from build123d import *

# Parameters (mm, degrees)
SKETCH1_W           = 42.3
SKETCH1_H           = 60
SKETCH1_R           = 8
SKETCH1_W_2         = 4
SKETCH1_H_2         = 5.4
BOSS_EXTRUDE1_DEPTH = 3.175
SKETCH2_R           = 7.95936
BOSS_EXTRUDE3_DEPTH = 3.175
SKETCH3_R           = 7.91872
BOSS_EXTRUDE4_DEPTH = 3.175


with BuildPart() as part:
    # Sketch1 → Boss-Extrude1 (new body)
    with BuildSketch(Plane.XY):
        Rectangle(SKETCH1_W, SKETCH1_H)
        Circle(SKETCH1_R, mode=Mode.SUBTRACT)
        with Locations((0, -32.7)):
            Rectangle(SKETCH1_W_2, SKETCH1_H_2)
        with Locations((-11.5, -32.7)):
            Rectangle(SKETCH1_W_2, SKETCH1_H_2)
        with Locations((11.5, -32.7)):
            Rectangle(SKETCH1_W_2, SKETCH1_H_2)
    extrude(amount=BOSS_EXTRUDE1_DEPTH)

    # Sketch2 → Boss-Extrude3 (add)
    with BuildSketch(Plane.XY.offset(3.175)):
        Polygon((21.19064, -30.04064), (21.19064, 30.04064), (-21.19064, 30.04064), (-21.19064, -30.04064), (-13.54064, -30.04064), (-13.54064, -35.44064), (-9.45936, -35.44064), (-9.45936, -30.04064), (-2.04064, -30.04064), (-2.04064, -35.44064), (2.04064, -35.44064), (2.04064, -30.04064), (9.45936, -30.04064), (9.45936, -35.44064), (13.54064, -35.44064), (13.54064, -30.04064), align=None)
        Circle(SKETCH2_R, mode=Mode.SUBTRACT)
    extrude(amount=-BOSS_EXTRUDE3_DEPTH)

    # Sketch3 → Boss-Extrude4 (add)
    with BuildSketch(Plane.XY.offset(3.175)):
        Polygon((-21.23128, 30.08128), (-21.23128, -30.08128), (-13.58128, -30.08128), (-13.58128, -35.48128), (-9.41872, -35.48128), (-9.41872, -30.08128), (-2.08128, -30.08128), (-2.08128, -35.48128), (2.08128, -35.48128), (2.08128, -30.08128), (9.41872, -30.08128), (9.41872, -35.48128), (13.58128, -35.48128), (13.58128, -30.08128), (21.23128, -30.08128), (21.23128, 30.08128), align=None)
        Circle(SKETCH3_R, mode=Mode.SUBTRACT)
    extrude(amount=-BOSS_EXTRUDE4_DEPTH)


solid = part.part
Model file for the job. Use its own axes, mm. A direction names the side the tool comes from. Coordinates: 2 decimals unless noted, no trailing zeros. Order: outer loops, then holes, each group sorted by start corner. A loop starts at its lowest first (then second) coordinate and runs counter-clockwise, first axis right, second up. Notation, with made-up numbers: (45, 53) -> (57, 53) arc R23 ccw to (57, 82) -> close; hole circle Ø7 at (45.25, 10). An arc over 180 degrees is marked (long way). Return JSON: item names as keys, results as strings. Group by question number.
Item 1: Tool access for faces 5 (the flat face through (13.581, -33, 2)), 6 (the flat face through (-10, -2, 3.175)), 7 (the flat face through (2.081, -33, 2)), 8 (the flat face through (-17, -30.081, 2)): list every direction of +Z, -Z, +X, -X, +Y, -Y with a clear straight run to the whole face (end or side of a thin tool).
Item 2: Flat gauge pins, fed straight in: P1, Ø1.6, axis at x = 19, z = 1, coming from the -Y side; P2, Ø1.6, axis at y = -33.5, z = 1.5, coming from the -X side. Where does each tip first touch, or does it go through?
Item 3: Saw through at B-B on z = 1.85. Write the cut outline in (x, y).
Item 4: Pull direction X, two halves, no side cores. Call faces 1 (the flat face through (-21.231, 0, 2)), 2 (the flat face through (0, -35.481, 2)), 3 (the flat face through (6, -30.081, 2)), 4 (the flat face through (21.231, 0, 2)): pulls with the +X half, pulls with the -X half, needs draft (parallel to the pull), parting line crosses it, or undercut.
Item 5: Wall check: line 1 along Y through (x, z) = (0, 1.3); line 2 along X through (y, z) = (3, 1.45); line 3 along X through (y, z) = (-4, 1.7). Give the ranges that are in metal, low to high. Write a range as [from, to].
Item 6: Saw through at A-A on x = 0. Write the cut outline in (y, z) (3 decimals).
Item 7: Saw through at C-C on y = 0. Write the cut outline in (x, z) (3 decimals).
Values found:
{
 "1": {"face 5": "+Z, -Z, +X, -Y", "face 6": "+Z, +X, -X, +Y, -Y", "face 7": "+Z, -Z, -Y", "face 8": "+Z, -Z, -X, -Y"},
 "2": {"P1": "stops at y = -30.08", "P2": "stops at x = -13.58"},
 "3": {"outline": "(-21.23, -30.08) -> (-13.58, -30.08) -> (-13.58, -35.48) -> (-9.42, -35.48) -> (-9.42, -30.08) -> (-2.08, -30.08) -> (-2.08, -35.48) -> (2.08, -35.48) -> (2.08, -30.08) -> (9.42, -30.08) -> (9.42, -35.48) -> (13.58, -35.48) -> (13.58, -30.08) -> (21.23, -30.08) -> (21.23, 30.08) -> (-21.23, 30.08) -> close; hole circle Ø15.84 at (0, 0)"},
 "4": {"face 1": "pulls with the -X half", "face 2": "needs draft", "face 3": "undercut", "face 4": "pulls with the +X half"},
 "5": {"line 1": "y = [-35.48, -7.92], [7.92, 30.08]", "line 2": "x = [-21.23, -7.33], [7.33, 21.23]", "line 3": "x = [-21.23, -6.83], [6.83, 21.23]"},
 "6": {"outline": "(-35.481, 0) -> (-7.919, 0) -> (-7.919, 3.175) -> (-35.481, 3.175) -> close; (7.919, 0) -> (30.081, 0) -> (30.081, 3.175) -> (7.919, 3.175) -> close"},
 "7": {"outline": "(-21.231, 0) -> (-7.919, 0) -> (-7.919, 3.175) -> (-21.231, 3.175) -> close; (7.919, 0) -> (21.231, 0) -> (21.231, 3.175) -> (7.919, 3.175) -> close"}
}
